```python
from build123d import *

# Parameters (mm, degrees)
SKETCH_R      = 15
SKETCH_R_2    = 2
PAD_DEPTH     = 9
SKETCH001_R   = 5
SKETCH001_R_2 = 2
PAD001_DEPTH  = 1


with BuildPart() as pad:
    # Sketch → Pad (new body)
    with BuildSketch(Plane.XZ):
        Circle(SKETCH_R)
        Circle(SKETCH_R_2, mode=Mode.SUBTRACT)
    extrude(amount=PAD_DEPTH)


with BuildPart() as fusion:
    # Pad001 base: copy of Pad
    add(pad.part)

    # Sketch001 → Pad001 (new body)
    with BuildSketch(Plane.XZ.offset(9)):
        Circle(SKETCH001_R)
        Circle(SKETCH001_R_2, mode=Mode.SUBTRACT)
    extrude(amount=PAD001_DEPTH)

    # Fusion: union Pad
    add(pad.part)


solid = fusion.part
```
The model under review builds one solid part; all positions refer to its coordinate system, in mm. A direction names the side the tool comes from. Coordinates: 2 decimals unless noted, no trailing zeros. Write each loop counter-clockwise with the first axis right and the second up, starting at its lowest first coordinate (ties: lowest second). Pieces come first, ordered by that corner, then holes. Notation, with made-up numbers: (-8, 20.5) -> (12, 20.5) arc R19 cw to (12, 42.5) -> close; hole circle Ø6 at (73, 42). An arc over 180 degrees is marked (long way). One line per item, written item: value. Start each with the question number.
Q1. Add section A-A, the plane x = 0. Give the boundary of the cut face in (y, z), then the cut area to 3 significant figures.
Q2. Add section D-D, the plane x = -3.5. Give the boundary of the cut face in (y, z), then the cut area to 3 significant figures.
Q3. Add section C-C, the plane y = -7.75. Give the boundary of the cut face in (x, z).
Q4. The part is to be moulded in two halves that separate along Z. For faces 1 (the face through (-14.985, -4.437, 0.66)), 2 (the face through (0, -5, -2)), 3 (the face through (-4, -9, 4)), say which applies: +Z half, -Z half, draft (parallel to the pull), parting line (faces both ways), or undercut.
Q5. Add section B-B, the plane z = 0. Give the boundary of the cut face in (x, y), then the cut area to 3 significant figures.
Q6. Clearance check with flat-ended pins moving along their axes: P1, Ø5, axis at y = -2, z = -9, coming from the -X side; P2, Ø2, axis at x = 11.5, y = -2, coming from the +Z side; P3, Ø2, axis at x = -9.5, y = -6, coming from the -Z side. State where each tip first meets the part, or that it passes through.
Q7. To check wall thickness, follow probe 1 along Z at (x, y) = (0, -4.5); probe 2 along Y at (x, z) = (7.5, -6.5); probe 3 along Z at (x, y) = (-1, -6.25). State the ranges of each line that lie inside material, in increasing order.
Q8. For faces 4 (the face through (3, 0, 0)), 5 (the face through (-1.08, -9.49, -4.88)), list the 3-axis set-ups (+Z, -Z, +X, -X, +Y, -Y) from which the entire face can be reached by the end or side of a thin tool; tool diameter is ignored.
Response:
1. outline: (-10, -5) -> (-9, -5) -> (-9, -15) -> (0, -15) -> (0, -2) -> (-10, -2) -> close; (-10, 2) -> (0, 2) -> (0, 15) -> (-9, 15) -> (-9, 5) -> (-10, 5) -> close
1. area: 240 mm²
2. outline: (-10, -3.57) -> (-9, -3.57) -> (-9, -14.59) -> (0, -14.59) -> (0, 14.59) -> (-9, 14.59) -> (-9, 3.57) -> (-10, 3.57) -> close
2. area: 270 mm²
3. outline: circle Ø30 at (0, 0); hole circle Ø4 at (0, 0)
4. face 1: parting line
4. face 2: undercut
4. face 3: draft
5. outline: (-15, -9) -> (-5, -9) -> (-5, -10) -> (-2, -10) -> (-2, 0) -> (-15, 0) -> close; (2, -10) -> (5, -10) -> (5, -9) -> (15, -9) -> (15, 0) -> (2, 0) -> close
5. area: 240 mm²
6. P1: x = -13.52
6. P2: z = 10.71
6. P3: z = -12.36
7. probe 1: -15 to -2, 2 to 15
7. probe 2: -9 to 0
7. probe 3: -14.97 to -1.73, 1.73 to 14.97
8. face 4: +Z, -Z, +X, -X, +Y
8. face 5: -Y
